Verification items for the finished model (mm, model axes). Give positions to 0.01 mm unless a question says otherwise; leave off trailing zeros. Order: outer loops, then holes, each group sorted by start corner. A loop starts at its lowest first (then second) coordinate and runs counter-clockwise, first axis right, second up. Notation, with made-up numbers: (5, 29.5) -> (29, 29.5) arc R11 ccw to (29, 46.5) -> close; hole circle Ø3 at (81.25, 57). An arc over 180 degrees is marked (long way). Write each question's results on one line, items separated by ' | '. Start each with the question number.
1. Cross-section at B-B, the plane y = 70. Enter the section's corners in (x, z), then the cut area to 3 significant figures.
2. Material ranges on L1, parallel to Z at x = 41, y = 98.5; L2, parallel to X at y = -105.5, z = 2.45; L3, parallel to X at y = 95, z = 3.6, recorded low to high. Write a range as from..to.
3. Cross-section at A-A, the plane y = -54.5. Enter the section's corners in (x, z).
4. Depth check by flat-ended pin: pin 1 Ø4.5 at (x, y) = (-41, 95) entering from -Z; pin 2 Ø10 at (x, y) = (40.1, 95) entering from +Z; pin 3 Ø1.5 at (x, z) = (-32.5, 4) entering from -Y; pin 4 Ø1.5 at (y, z) = (28, 2.5) entering from +X. Enter the tip coordinate at first touch or a pass-through.
Autodesk Fusion 360 part; units mm, degrees
sketch "Sketch2" plane through (0, 0, 0) normal (0, 0, 1) x (1, 0, 0)
  line L0 (-41, 95) -> (40.1, 95) construction
  circle A0 centre (-41, 95) radius 1.75
  circle A1 centre (40.1, 95) radius 1.75
  line L1 (-32.1418, -106.2761) -> (29.9104, -106.2761) construction
  circle A2 centre (-32.1418, -106.2761) radius 1.75
  circle A3 centre (29.9104, -106.2761) radius 1.75
  line L2 (0, 125.7) -> (-30.2729, 125.7)
  line L3 (0, -124.4) -> (-26.7617, -124.4)
  line L4 (-40.5, -110.5) -> (-50.5, 104.7)
  arc A4 (-40.5, -110.5) -> (-26.7617, -124.4) centre (-25.9132, -109.8222) ccw
  arc A5 (-45.3008, 119.9335) -> (-50.5, 104.7) centre (-28.5694, 105.7191) ccw
  arc A6 (-30.2729, 125.7) -> (-45.3008, 119.9335) centre (-30.2729, 103.2348) ccw
  arc A7 (43.3008, 119.9335) -> (28.2729, 125.7) centre (28.2729, 103.2348) ccw
  arc A8 (48.5, 104.7) -> (43.3008, 119.9335) centre (26.5694, 105.7191) ccw
  line L5 (38.5, -110.5) -> (48.5, 104.7)
  arc A9 (24.7617, -124.4) -> (38.5, -110.5) centre (23.9132, -109.8222) ccw
  line L6 (0, 125.7) -> (28.2729, 125.7)
  line L7 (0, -124.4) -> (24.7617, -124.4)
  circle A10 centre (-41, 95) radius 3.75
  circle A11 centre (-41, 95) radius 3.75
  circle A12 centre (40.1, 95) radius 3.75
  circle A13 centre (-32.1418, -106.2761) radius 3.75
  circle A14 centre (29.9104, -106.2761) radius 3.75
  dimension "d1" = 3.5
  dimension "d2" = 62.0522
  dimension "d3" = 7.5
  dimension "d4" = 7.5
extrude "Extrude1" add sketch "Sketch2" along normal blind 5 contours L2 L3 L4 A4 A5 A6 A7 A8 L5 A9 L6 L7 | A10 A11 | A12 | A13 | A14
extrude "Extrude2" cut sketch "Sketch2" along normal blind 2.5 contours A10 A11 | A12 | A13 | A14
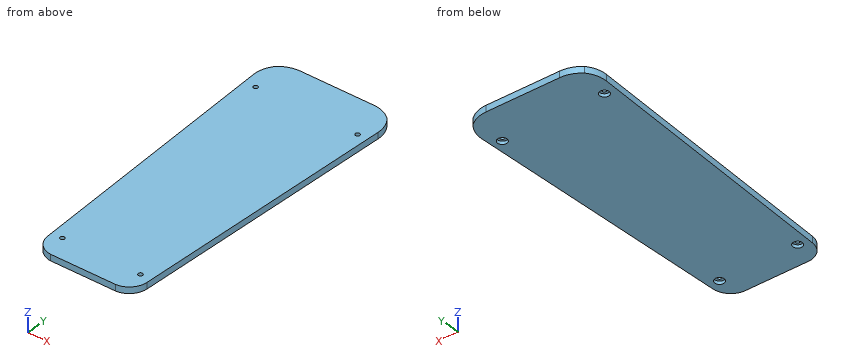
Results below:
1) outline: (-48.89, 0) -> (46.89, 0) -> (46.89, 5) -> (-48.89, 5) -> close | area: 479 mm²
2) L1: z = 2.5..5 | L2: x = -40.73..-35.81, -28.47..26.24, 33.58..38.73 | L3: x = -50.05..-42.75, -39.25..38.35, 41.85..48.05
3) outline: (-43.1, 0) -> (41.1, 0) -> (41.1, 5) -> (-43.1, 5) -> close
4) pin 1: stops at z = 2.5 | pin 2: stops at z = 5 | pin 3: stops at y = -123.21 | pin 4: stops at x = 44.97
